```python
from build123d import *

# Parameters (mm, degrees)
F0_W     = 76.2
F0_H     = 101.6
F0_W_2   = 69.85
F0_H_2   = 95.25
F1_DEPTH = 914.4
F2_R     = 9.525
F3_DEPTH = 76.2
F4_W     = 69.85
F4_H     = 114.3
F5_DEPTH = 3.175
F6_R     = 25.4
F6_R_2   = 20.6375
F7_DEPTH = 14.2875
F8_R     = 25.4
F8_R_2   = 20.6375
F9_DEPTH = 14.2875


with BuildPart() as f1:
    # F0 (on Front) → F1 (new body)
    with BuildSketch(Plane.XZ):
        with Locations((38.1, 50.8)):
            Rectangle(F0_W, F0_H)
        with Locations((38.1, 50.8)):
            Rectangle(F0_W_2, F0_H_2, mode=Mode.SUBTRACT)
    extrude(amount=F1_DEPTH)

    # F2 (on Right) → F3 (cut)
    with BuildSketch(Plane.YZ):
        with Locations((-850.9, 38.1)):
            Circle(F2_R)
        with Locations((-63.5, 38.1)):
            Circle(F2_R)
    extrude(amount=F3_DEPTH, mode=Mode.SUBTRACT)

    # F4 (on Top) → F5 (cut)
    with BuildSketch(Plane.XY):
        with Locations((38.1, -857.25)):
            Rectangle(F4_W, F4_H)
        with Locations((38.1, -57.15)):
            Rectangle(F4_W, F4_H)
    extrude(amount=F5_DEPTH, mode=Mode.SUBTRACT)

    # F6 (on face) → F7 (join)
    with BuildSketch(Plane.YZ.offset(76.2)):
        with Locations((-850.9, 38.1)):
            Circle(F6_R)
        with Locations((-850.9, 38.1)):
            Circle(F6_R_2, mode=Mode.SUBTRACT)
        with Locations((-63.5, 38.1)):
            Circle(F6_R)
        with Locations((-63.5, 38.1)):
            Circle(F6_R_2, mode=Mode.SUBTRACT)
    extrude(amount=F7_DEPTH)

    # F8 (on face) → F9 (join)
    with BuildSketch(Plane(origin=(0, 0, 0), x_dir=(0, -1, 0), z_dir=(-1, 0, 0))):
        with Locations((63.5, 38.1)):
            Circle(F8_R)
        with Locations((63.5, 38.1)):
            Circle(F8_R_2, mode=Mode.SUBTRACT)
        with Locations((850.9, 38.1)):
            Circle(F8_R)
        with Locations((850.9, 38.1)):
            Circle(F8_R_2, mode=Mode.SUBTRACT)
    extrude(amount=F9_DEPTH)


solid = f1.part
```
Could you check a few things on this model? Use its own coordinates, in mm. A direction names the side the tool comes from. Round coordinates to 2 decimals unless told otherwise and drop trailing zeros. Loops run counter-clockwise (first coordinate to the right, second up) from the corner with the lowest first, then second, coordinate; pieces in that order, holes last. Notation, with made-up numbers: M -29,27.5 L 22,27.5 A20 cw 22,52.5 Z; hole C 27,28 d10. An arc over 180 degrees is marked long. Write item = value, one per line.
1. Thinking about a two-plate mould opening in Z: for faces 1 (the face through (76.2, -451, 50)), 2 (the face through (0, -855, 47)), 3 (the face through (-7.044, -75.221, 15.566)), which applies, +Z half, -Z half, draft (parallel to the pull), parting line (faces both ways), or undercut?
Results below:
face_1 = draft
face_2 = undercut
face_3 = parting line
2. I want a section at A-A, the plane x = 32. Write out the boundary of the cut face in (y, z) (3 decimals).
Results below:
outline = M -914.4,98.425 L 0,98.425 L 0,101.6 L -914.4,101.6 Z; M -800.1,0 L -114.3,0 L -114.3,3.175 L -800.1,3.175 Z
3. I want a section at B-B, the plane y = -63.5. Count the separate pieces of the cut face and the enclosed holes in it, and give its area (3 significant figures).
Results below:
separate_pieces = 3
enclosed_holes = 0
area = 1,020 mm²
4. Will these pins go through, and if not, where does the flat tip stop? P1, Ø25, axis at y = -63.5, z = 38.1, coming from the +X side; P2, Ø1, axis at y = -503, z = 90.5, coming from the -X side; P3, Ø11.5, axis at y = -63.5, z = 38.1, coming from the -X side; P4, Ø1.6, axis at x = 37, z = 1.5, coming from the -Y side.
Results below:
P1 = 76.2
P2 = 0
P3 = through
P4 = -800.1
5. Which directions (+Z, -Z, +X, -X, +Y, -Y) give clear straight access to the entire face, cutting with the end or side of a thin tool? Please do faces 4 (the face through (38, -451, 0)), 5 (the face through (83.244, -831.216, 44.299)), 6 (the face through (-7.04, -860.42, 19.79)), 7 (the face through (38, -452, 3.175)).
Results below:
face_4 = -Z, +X, -X, +Y, -Y
face_5 = +X
face_6 = -X
face_7 = +Y, -Y
6. I need wall thicknesses on probe 1 along Y at (x, z) = (0.75, 38.1) (3 decimals); probe 2 along X at (y, z) = (-453.5, 12) (3 decimals); probe 3 along Z at (x, y) = (2, -850). Which ranges of each line are inside material? Lowest first, please.
Results below:
probe_1 = -914.4 to -860.425, -841.375 to -73.025, -53.975 to 0
probe_2 = 0 to 3.175, 73.025 to 76.2
probe_3 = 0 to 28.62, 47.58 to 101.6
7. I want a section at D-D, the plane y = -631. Write out the boundary of the cut face in (x, z) (3 decimals), and give its area (3 significant figures).
Results below:
outline = M 0,0 L 76.2,0 L 76.2,101.6 L 0,101.6 Z; hole M 3.175,3.175 L 73.025,3.175 L 73.025,98.425 L 3.175,98.425 Z
area = 1,090 mm²
